```python
from build123d import *

# Parameters (mm, degrees)
SKETCH2_R           = 50
SKETCH2_R_2         = 47
BOSS_EXTRUDE2_DEPTH = 10
SKETCH4_W           = 16.15
SKETCH4_H           = 16.43
CUT_EXTRUDE1_DEPTH  = 10
SKETCH3_R           = 40
SKETCH3_R_2         = 37
BOSS_EXTRUDE3_DEPTH = 10


with BuildPart() as part:
    # Sketch1 → Revolve1 (revolve)
    with BuildSketch(Plane(origin=(0, 0, 0), x_dir=(0, 0, -1), z_dir=(1, 0, 0)), mode=Mode.PRIVATE) as revolve1_sk:
        Polygon((0, 0), (3, 0), (3, 47), (247, 37.24), (247, 0), (250, 0), (250, 40), (0, 50), align=None)
    revolve(revolve1_sk.sketch.rotate(Axis((0, 0, 0), (0, 0, -1)), 90), axis=Axis((0, 0, 0), (0, 0, -1)))

    # Sketch2 → Boss-Extrude2 (add)
    with BuildSketch(Plane.XY):
        Circle(SKETCH2_R)
        Circle(SKETCH2_R_2, mode=Mode.SUBTRACT)
    extrude(amount=BOSS_EXTRUDE2_DEPTH)

    # Sketch4 → Cut-Extrude1 (cut)
    with BuildSketch(Plane.XY):
        Rectangle(SKETCH4_W, SKETCH4_H)
    extrude(amount=-CUT_EXTRUDE1_DEPTH, mode=Mode.SUBTRACT)

    # Sketch3 → Boss-Extrude3 (add)
    with BuildSketch(Plane.XY.offset(-250)):
        Circle(SKETCH3_R)
        Circle(SKETCH3_R_2, mode=Mode.SUBTRACT)
    extrude(amount=-BOSS_EXTRUDE3_DEPTH)


solid = part.part
```
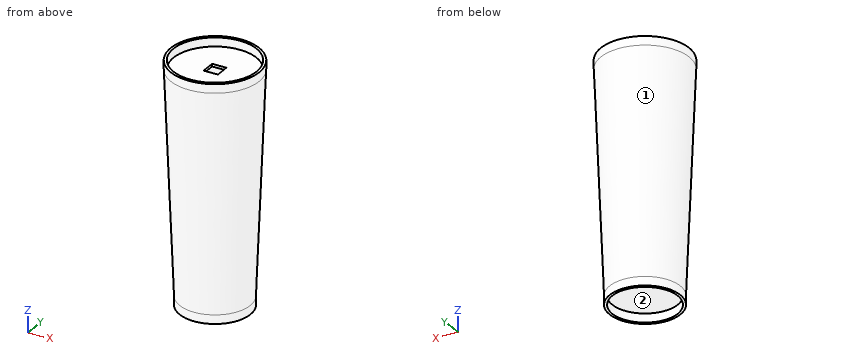
Verification items for the finished model (mm, model axes). Face numbers are marked on the shaded views. Coordinates: 2 decimals unless noted, no trailing zeros. Loops run counter-clockwise (first coordinate to the right, second up) from the corner with the lowest first, then second, coordinate; pieces in that order, holes last. Notation, with made-up numbers: (65.5, -18.5) -> (86.5, -18.5) arc R16 cw to (86.5, 3.5) -> close; hole circle Ø10 at (8, 48.25). An arc over 180 degrees is marked (long way). Answer in a Markdown table with one row per item. Add a question column.
1. Section check B-B, the plane z = -121. Enter the section's corners in (x, y), then the cut area to 3 significant figures.
2. Section check D-D, the plane z = -218.5. Enter the section's corners in (x, y).
3. Draft check along Y on the marked faces 1 and 2. Enter one of: +Y half, -Y half, draft (parallel to the pull), parting line (faces both ways), or undercut.
4. Material ranges on probe 1 along Z at (x, y) = (-25, -0.5); probe 2 along Y at (x, z) = (0, 5); probe 3 along Y at (x, z) = (0, -252.25), recorded low to high. Write a range as [from, to].
5. Section check A-A, the plane x = 0. Enter the section's corners in (y, z) (3 decimals).
6. Depth check by flat-ended pin: P1, Ø2.5, axis at y = 0.5, z = -2, coming from the -X side; P2, Ø1.5, axis at x = 0.5, z = -1, coming from the -Y side; P3, Ø5, axis at x = -21.5, z = -78.5, coming from the +Y side. Enter the tip coordinate at first touch or a pass-through.
7. Section check C-C, the plane y = 0. Enter the section's corners in (x, z) (3 decimals).
Derived:
| question | item | result |
|---|---|---|
| 1 | outline | circle Ø90.32 at (0, 0); hole circle Ø84.56 at (0, 0) |
| 1 | area | 791 mm² |
| 2 | outline | circle Ø82.52 at (0, 0); hole circle Ø76.76 at (0, 0) |
| 3 | face 1 | parting line |
| 3 | face 2 | undercut |
| 4 | probe 1 | z = [-250, -247], [-3, 0] |
| 4 | probe 2 | y = [-50, -47], [47, 50] |
| 4 | probe 3 | y = [-40, -37], [37, 40] |
| 5 | outline | (-50, 0) -> (-40, -250) -> (-40, -260) -> (-37, -260) -> (-37, -250) -> (37, -250) -> (37, -260) -> (40, -260) -> (40, -250) -> (50, 0) -> (50, 10) -> (47, 10) -> (47, 0) -> (8.215, 0) -> (8.215, -3) -> (47, -3) -> (37.24, -247) -> (-37.24, -247) -> (-47, -3) -> (-8.215, -3) -> (-8.215, 0) -> (-47, 0) -> (-47, 10) -> (-50, 10) -> close |
| 6 | P1 | stops at x = -49.97 |
| 6 | P2 | stops at y = -49.99 |
| 6 | P3 | stops at y = 42.84 |
| 7 | outline | (-50, 0) -> (-40, -250) -> (-40, -260) -> (-37, -260) -> (-37, -250) -> (37, -250) -> (37, -260) -> (40, -260) -> (40, -250) -> (50, 0) -> (50, 10) -> (47, 10) -> (47, 0) -> (8.075, 0) -> (8.075, -3) -> (47, -3) -> (37.24, -247) -> (-37.24, -247) -> (-47, -3) -> (-8.075, -3) -> (-8.075, 0) -> (-47, 0) -> (-47, 10) -> (-50, 10) -> close |
